```python
from build123d import *

# Parameters (mm, degrees)
SKETCH_1_W          = 70
SKETCH_1_H          = 40
EXTRUDE_1_DEPTH     = 40
SKETCH_2_W          = 20
SKETCH_2_H          = 20
CUT_EXTRUDE_1_DEPTH = 10
SKETCH_3_W          = 40
SKETCH_3_H          = 20
CUT_EXTRUDE_2_DEPTH = 20


with BuildPart() as part:
    # 스케치1 → 보스-돌출1 (new body)
    with BuildSketch(Plane(origin=(0, 0, 0), x_dir=(1, 0, 0), z_dir=(0, 1, 0))):
        with Locations((35, 20)):
            Rectangle(SKETCH_1_W, SKETCH_1_H)
    extrude(amount=EXTRUDE_1_DEPTH)

    # 스케치2 → 컷-돌출1 (cut)
    with BuildSketch(Plane(origin=(0, 40, 0), x_dir=(1, 0, 0), z_dir=(0, 1, 0))):
        with Locations((60, 30)):
            Rectangle(SKETCH_2_W, SKETCH_2_H)
    extrude(amount=-CUT_EXTRUDE_1_DEPTH, mode=Mode.SUBTRACT)

    # 스케치3 → 컷-돌출2 (cut)
    with BuildSketch(Plane(origin=(0, 40, 0), x_dir=(1, 0, 0), z_dir=(0, 1, 0))):
        with Locations((50, 10)):
            Rectangle(SKETCH_3_W, SKETCH_3_H)
    extrude(amount=-CUT_EXTRUDE_2_DEPTH, mode=Mode.SUBTRACT)


solid = part.part
```
Geometry check sheet. Reference: the model listing, model coordinates, mm. A direction names the side the tool comes from. Round coordinates to 2 decimals unless told otherwise and drop trailing zeros. Order: outer loops, then holes, each group sorted by start corner. A loop starts at its lowest first (then second) coordinate and runs counter-clockwise, first axis right, second up. Notation, with made-up numbers: (16.5, 52) -> (22.5, 52) arc R26 ccw to (22.5, 88) -> close; hole circle Ø7 at (46, -5.75). An arc over 180 degrees is marked (long way). Return JSON: item names as keys, results as strings. Group by question number.
Q1. Material ranges on probe 1 along X at (y, z) = (27.5, -5.5); probe 2 along Z at (x, y) = (61, 29); probe 3 along Y at (x, z) = (64.5, -13.5), recorded low to high. Write a range as from..to.
Q2. Gauge pin test, flat ends, axial feed: pin 1 (16 mm diameter, centred on x = 43.5, z = -10, fed in from +Y); pin 2 (22 mm diameter, centred on x = 63, z = -29.5, fed in from +Y); pin 3 (10 mm diameter, centred on y = 26, z = -10, fed in from +X). Record the tip position at first contact, or that the pin passes through.
Q3. Tool access check on faces 1 (the flat face through (60, 30, -30)), 2 (the flat face through (70, 11, -20)), 3 (the flat face through (45, 28, -20)). Record the directions out of +Z, -Z, +X, -X, +Y, -Y that give a thin tool (end or side, any length) a straight path to the whole face; none if there is none.
Q4. Section check B-B, the plane z = -5. Record the boundary of the cut face in (x, y), plus the area to 3 significant figures.
Q5. Section check A-A, the plane x = 58.5. Record the boundary of the cut face in (y, z).
Numbers:
{
 "1": {"probe 1": "0..30", "probe 2": "-40..-20", "probe 3": "0..20"},
 "2": {"pin 1": "y = 20", "pin 2": "y = 30", "pin 3": "x = 30"},
 "3": {"face 1": "+Z, -Z, +X, +Y", "face 2": "+Z, -Z, +X, +Y, -Y", "face 3": "+Z, +X, +Y"},
 "4": {"outline": "(0, 0) -> (70, 0) -> (70, 20) -> (30, 20) -> (30, 40) -> (0, 40) -> close", "area": "2,000 mm^2"},
 "5": {"outline": "(0, -40) -> (30, -40) -> (30, -20) -> (20, -20) -> (20, 0) -> (0, 0) -> close"}
}
